from build123d import *

# Parameters (mm, degrees)
F0_R     = 12.7
F1_DEPTH = 6.35


with BuildPart() as f1:
    # F0 (on Top) → F1 (new body)
    with BuildSketch(Plane.XY):
        with BuildLine():
            ThreePointArc((-57.94375, 25.976370723), (-52.8530385151, 35.1966805213), (-46.3083103346, 43.4487099228))
            ThreePointArc((-46.3083103346, 43.4487099228), (-59.3557480022, 34.5595657373), (-74.8865363941, 31.7228200726))
            ThreePointArc((-74.8865363941, 31.7228200726), (-66.002017715, 30.0676513435), (-57.94375, 25.976370723))
        make_face()
        with BuildLine():
            ThreePointArc((-44.45, 0), (-48.024670033, 14.636026826), (-57.94375, 25.976370723))
            ThreePointArc((-57.94375, 25.976370723), (-62.0954029096, 13.2819779212), (-63.5, 0))
            ThreePointArc((-63.5, 0), (-62.0954029096, -13.2819779212), (-57.94375, -25.976370723))
            ThreePointArc((-57.94375, -25.976370723), (-48.024670033, -14.636026826), (-44.45, 0))
        make_face()
        with BuildLine():
            ThreePointArc((-63.5, 0), (-62.0954029096, 13.2819779212), (-57.94375, 25.976370723))
            ThreePointArc((-57.94375, 25.976370723), (-66.002017715, 30.0676513435), (-74.8865363941, 31.7228200726))
            ThreePointArc((-74.8865363941, 31.7228200726), (-75.1174911921, 31.7299983006), (-75.3483982089, 31.7385770694))
            ThreePointArc((-75.3483982089, 31.7385770694), (-107.95, 0), (-75.3483982089, -31.7385770694))
            ThreePointArc((-75.3483982089, -31.7385770694), (-75.1174911921, -31.7299983006), (-74.8865363941, -31.7228200726))
            ThreePointArc((-74.8865363941, -31.7228200726), (-66.002017715, -30.0676513435), (-57.94375, -25.976370723))
            ThreePointArc((-57.94375, -25.976370723), (-62.0954029096, -13.2819779212), (-63.5, 0))
        make_face()
        with Locations((-76.2, 0)):
            Circle(F0_R, mode=Mode.SUBTRACT)
        with BuildLine():
            ThreePointArc((57.94375, -25.976370723), (48.024670033, -14.636026826), (44.45, 0))
            ThreePointArc((44.45, 0), (0, -44.45), (-44.45, 0))
            ThreePointArc((-44.45, 0), (-48.024670033, -14.636026826), (-57.94375, -25.976370723))
            ThreePointArc((-57.94375, -25.976370723), (-52.8530385151, -35.1966805213), (-46.3083103346, -43.4487099228))
            ThreePointArc((-46.3083103346, -43.4487099228), (0, -63.5), (46.3083103346, -43.4487099228))
            ThreePointArc((46.3083103346, -43.4487099228), (52.8530385151, -35.1966805213), (57.94375, -25.976370723))
        make_face()
        with BuildLine():
            ThreePointArc((-46.3083103346, -43.4487099228), (-52.8530385151, -35.1966805213), (-57.94375, -25.976370723))
            ThreePointArc((-57.94375, -25.976370723), (-66.002017715, -30.0676513435), (-74.8865363941, -31.7228200726))
            ThreePointArc((-74.8865363941, -31.7228200726), (-59.3557480022, -34.5595657373), (-46.3083103346, -43.4487099228))
        make_face()
        with BuildLine():
            ThreePointArc((57.94375, 25.976370723), (52.8530385151, 35.1966805213), (46.3083103346, 43.4487099228))
            ThreePointArc((46.3083103346, 43.4487099228), (0, 63.5), (-46.3083103346, 43.4487099228))
            ThreePointArc((-46.3083103346, 43.4487099228), (-52.8530385151, 35.1966805213), (-57.94375, 25.976370723))
            ThreePointArc((-57.94375, 25.976370723), (-48.024670033, 14.636026826), (-44.45, 0))
            ThreePointArc((-44.45, 0), (0, 44.45), (44.45, 0))
            ThreePointArc((44.45, 0), (48.024670033, 14.636026826), (57.94375, 25.976370723))
        make_face()
        with BuildLine():
            ThreePointArc((63.5, 0), (62.0954029096, 13.2819779212), (57.94375, 25.976370723))
            ThreePointArc((57.94375, 25.976370723), (48.024670033, 14.636026826), (44.45, 0))
            ThreePointArc((44.45, 0), (48.024670033, -14.636026826), (57.94375, -25.976370723))
            ThreePointArc((57.94375, -25.976370723), (62.0954029096, -13.2819779212), (63.5, 0))
        make_face()
        with BuildLine():
            ThreePointArc((74.8865363941, 31.7228200726), (66.002017715, 30.0676513435), (57.94375, 25.976370723))
            ThreePointArc((57.94375, 25.976370723), (62.0954029096, 13.2819779212), (63.5, 0))
            ThreePointArc((63.5, 0), (62.0954029096, -13.2819779212), (57.94375, -25.976370723))
            ThreePointArc((57.94375, -25.976370723), (66.002017715, -30.0676513435), (74.8865363941, -31.7228200726))
            ThreePointArc((74.8865363941, -31.7228200726), (75.1174911921, -31.7299983006), (75.3483982089, -31.7385770694))
            ThreePointArc((75.3483982089, -31.7385770694), (98.3475071186, -22.7497346893), (107.95, 0))
            ThreePointArc((107.95, 0), (98.3475071186, 22.7497346893), (75.3483982089, 31.7385770694))
            ThreePointArc((75.3483982089, 31.7385770694), (75.1174911921, 31.7299983006), (74.8865363941, 31.7228200726))
        make_face()
        with BuildLine():
            ThreePointArc((88.9, 0), (76.2, -12.7), (63.5, 0))
            ThreePointArc((63.5, 0), (76.2, 12.7), (88.9, 0))
        make_face(mode=Mode.SUBTRACT)
        with BuildLine():
            ThreePointArc((74.8865363941, 31.7228200726), (59.3557480022, 34.5595657373), (46.3083103346, 43.4487099228))
            ThreePointArc((46.3083103346, 43.4487099228), (52.8530385151, 35.1966805213), (57.94375, 25.976370723))
            ThreePointArc((57.94375, 25.976370723), (66.002017715, 30.0676513435), (74.8865363941, 31.7228200726))
        make_face()
        with BuildLine():
            ThreePointArc((74.8865363941, -31.7228200726), (66.002017715, -30.0676513435), (57.94375, -25.976370723))
            ThreePointArc((57.94375, -25.976370723), (52.8530385151, -35.1966805213), (46.3083103346, -43.4487099228))
            ThreePointArc((46.3083103346, -43.4487099228), (59.3557480022, -34.5595657373), (74.8865363941, -31.7228200726))
        make_face()
    extrude(amount=F1_DEPTH)


solid = f1.part
Can you work these out from the model? Positions are in its coordinate system, mm. Coordinates: 2 decimals unless noted, no trailing zeros. Loops run counter-clockwise (first coordinate to the right, second up) from the corner with the lowest first, then second, coordinate; pieces in that order, holes last. Notation, with made-up numbers: (23, 55.25) - (82, 55.25) arc R22 ccw to (82, 84.25) - close; hole circle Ø2 at (20, 24). An arc over 180 degrees is marked (long way). Put each result on its own line as item: value. Start each with the question number.
Item 1: For pin 1 (3 mm diameter, centred on x = -43, z = 5, fed in from +Y); pin 2 (1.5 mm diameter, centred on x = 52, z = 5.5, fed in from +Y); pin 3 (3 mm diameter, centred on x = -48, z = 5.5, fed in from +Y), each with a flat end and sliding along its axis, tell me the tip position at first contact or that it passes through.
Item 2: Suppose I cut it at D-D (y = -9). Please give me the cut outline in (x, z), and give its area (3 significant figures).
Item 3: Suppose I cut it at C-C (z = 3.25). Please give me the cut outline in (x, y), and give its area (3 significant figures).
Item 4: Suppose I cut it at A-A (y = 18). Please give me the cut outline in (x, z).
Item 5: If we mould it in two halves opening along Y, with no side actions, what happens to faces 1 (the face through (-64.086, 3.815, 3.131)), 2 (the face through (46, 1, 6.35)), 3 (the face through (0.727, 63.496, 3.131))? For each: +Y half, -Y half, draft (parallel to the pull), parting line (faces both ways), or undercut.
Item 6: If I drill on line 1 along Y through (x, z) = (-76.2, 4.25); line 2 along Y through (x, z) = (0, 2.75); line 3 along X through (y, z) = (-3.5, 5.5), over which ranges is the centre line in solid material (lowest first)?
Item 7: Suppose I cut it at B-B (x = -16.5). Please give me the cut outline in (y, z).
Here are the results:
1. pin 1: y = 48.06
1. pin 2: y = 39.11
1. pin 3: y = 43.25
2. outline: (-106.65, 0) - (-85.16, 0) - (-85.16, 6.35) - (-106.65, 6.35) - close; (-67.24, 0) - (-43.53, 0) - (-43.53, 6.35) - (-67.24, 6.35) - close; (43.53, 0) - (67.24, 0) - (67.24, 6.35) - (43.53, 6.35) - close; (85.16, 0) - (106.65, 0) - (106.65, 6.35) - (85.16, 6.35) - close
2. area: 574 mm²
3. outline: (-75.35, -31.74) arc R38.1 cw to (-74.89, -31.72) arc R38.1 cw to (-46.31, -43.45) arc R63.5 ccw to (46.31, -43.45) arc R38.1 cw to (74.89, -31.72) arc R38.1 cw to (75.35, -31.74) arc R31.75 ccw (long way) to (75.35, 31.74) arc R38.1 cw to (74.89, 31.72) arc R38.1 cw to (46.31, 43.45) arc R63.5 ccw to (-46.31, 43.45) arc R38.1 cw to (-74.89, 31.72) arc R38.1 cw to (-75.35, 31.74) arc R31.75 ccw (long way) to start; hole circle Ø25.4 at (-76.2, 0); hole circle Ø88.9 at (0, 0); hole circle Ø25.4 at (76.2, 0)
3. area: 10,800 mm²
4. outline: (-102.35, 0) - (-40.64, 0) - (-40.64, 6.35) - (-102.35, 6.35) - close; (40.64, 0) - (102.35, 0) - (102.35, 6.35) - (40.64, 6.35) - close
5. face 1: undercut
5. face 2: draft
5. face 3: +Y half
6. line 1: -31.75 to -12.7, 12.7 to 31.75
6. line 2: -63.5 to -44.45, 44.45 to 63.5
6. line 3: -107.76 to -88.41, -63.99 to -44.31, 44.31 to 63.99, 88.41 to 107.76
7. outline: (-61.32, 0) - (-41.27, 0) - (-41.27, 6.35) - (-61.32, 6.35) - close; (41.27, 0) - (61.32, 0) - (61.32, 6.35) - (41.27, 6.35) - close
